```python
from build123d import *

# Parameters (mm, degrees)
SKETCH_1_R          = 6
EXTRUDE_1_DEPTH     = 10
SKETCH_2_R          = 2
CUT_EXTRUDE_1_DEPTH = 11
FILLET_1_R          = 1


with BuildPart() as part:
    # 草图1 → 凸台-拉伸1 (new body)
    with BuildSketch(Plane.XY):
        Circle(SKETCH_1_R)
    extrude(amount=EXTRUDE_1_DEPTH)

    # 草图2 → 切除-拉伸1 (cut, through all)
    with BuildSketch(Plane(origin=(0, 0, 0), x_dir=(-1, 0, 0), z_dir=(0, 0, -1))):
        Circle(SKETCH_2_R)
    extrude(amount=-CUT_EXTRUDE_1_DEPTH, mode=Mode.SUBTRACT)

    # 圆角1
    fillet_1_edges = [part.edges().sort_by_distance(p)[0] for p in [
        (-6, 0, 0),
        (-6, 0, 10),
    ]]
    fillet(fillet_1_edges, radius=FILLET_1_R)


solid = part.part
```
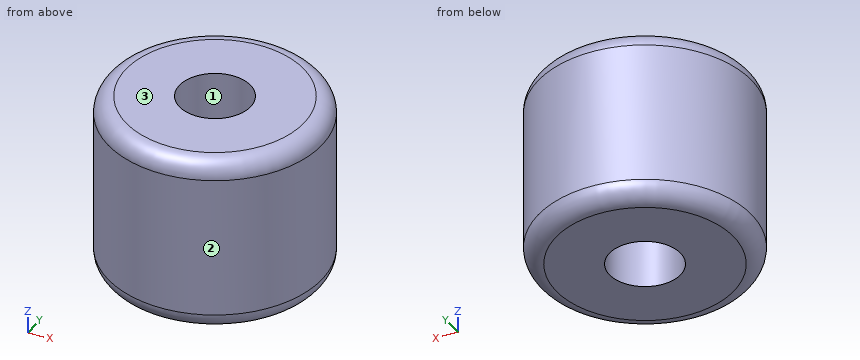
Could you check a few things on this model? Use its own coordinates, in mm. Face numbers are marked on the shaded views. Round coordinates to 2 decimals unless told otherwise and drop trailing zeros. Loops run counter-clockwise (first coordinate to the right, second up) from the corner with the lowest first, then second, coordinate; pieces in that order, holes last.
Q1. Thinking about a two-plate mould opening in X: for the marked faces 1, 2 and 3, which applies, pulls with the +X half, pulls with the -X half, needs draft (parallel to the pull), parting line crosses it, or undercut?
Q2. I want a section at C-C (z = 5.5). Write out the boundary of the cut face in (x, y), and give its area (3 significant figures).
Q3. For P1, Ø1.5, axis at x = 4.5, z = 5.5, coming from the +Y side, with a flat end and sliding along its axis, tell me the tip position at first contact or that it passes through.
Q4. Please list where these lines run through material, in increasing order: L1, parallel to Y at x = 0, z = 6.75; L2, parallel to Y at x = 0.5, z = 0.5; L3, parallel to X at y = 1, z = 1.5.
Q5. I want a section at A-A (x = 0). Write out the boundary of the cut face in (y, z), and give its area (3 significant figures).
Answer below:
1. face 1: undercut
1. face 2: parting line crosses it
1. face 3: needs draft
2. outline: circle Ø12 at (0, 0); hole circle Ø4 at (0, 0)
2. area: 101 mm2
3. P1: stops at y = 4.68
4. L1: y = -6 to -2, 2 to 6
4. L2: y = -5.84 to -1.94, 1.94 to 5.84
4. L3: x = -5.92 to -1.73, 1.73 to 5.92
5. outline: (-6, 1) arc R1 ccw to (-5, 0) - (-2, 0) - (-2, 10) - (-5, 10) arc R1 ccw to (-6, 9) - close; (2, 0) - (5, 0) arc R1 ccw to (6, 1) - (6, 9) arc R1 ccw to (5, 10) - (2, 10) - close
5. area: 79.1 mm2
